```python
from build123d import *

# Parameters (mm, degrees)
SKETCH1_R           = 37.5
BOSS_EXTRUDE1_DEPTH = 10
SKETCH3_R           = 1.5
CUT_EXTRUDE3_DEPTH  = 54.967582862
SKETCH4_R           = 5
CUT_EXTRUDE4_DEPTH  = 5
SKETCH5_R           = 1.5
CUT_EXTRUDE5_DEPTH  = 54.967582862
SKETCH6_R           = 3
CUT_EXTRUDE6_DEPTH  = 5
SKETCH8_R           = 3
CUT_EXTRUDE7_DEPTH  = 3
SKETCH9_R           = 10
CUT_EXTRUDE8_DEPTH  = 54.967582862


with BuildPart() as part:
    # Sketch1 → Boss-Extrude1 (new body)
    with BuildSketch(Plane(origin=(0, 0, 0), x_dir=(1, 0, 0), z_dir=(0, 1, 0))):
        with Locations(Location((0, 0, 0), (0, 0, 270))):
            Circle(SKETCH1_R)
    extrude(amount=BOSS_EXTRUDE1_DEPTH)

    # Sketch3 → Cut-Extrude3 (cut, through all)
    with BuildSketch(Plane(origin=(0, 10, 0), x_dir=(1, 0, 0), z_dir=(0, 1, 0))):
        with Locations(Location((0, 0, 0), (0, 0, 270))):
            Circle(SKETCH3_R)
    extrude(amount=-CUT_EXTRUDE3_DEPTH, mode=Mode.SUBTRACT)

    # Sketch4 → Cut-Extrude4 (cut)
    with BuildSketch(Plane.XZ):
        with Locations(Location((0, 0, 0), (0, 0, 270))):
            Circle(SKETCH4_R)
    extrude(amount=-CUT_EXTRUDE4_DEPTH, mode=Mode.SUBTRACT)

    # Sketch5 → Cut-Extrude5 (cut, through all)
    with BuildSketch(Plane(origin=(0, 10, 0), x_dir=(1, 0, 0), z_dir=(0, 1, 0))):
        with BuildLine():
            ThreePointArc((-18.854509148, 24.228237343), (-21.625950603, 24.261294568), (-19.689620544, 22.278214534))
            Line((-19.689620544, 22.278214534), (-20.247076251, 23.670781637))
            Line((-20.247076251, 23.670781637), (-18.854509148, 24.228237343))
        make_face()
        with BuildLine():
            Line((-20.247076251, 23.670781637), (-19.689620544, 22.278214534))
            ThreePointArc((-19.689620544, 22.278214534), (-19.004863797, 22.830003295), (-18.747076251, 23.670781637))
            ThreePointArc((-18.747076251, 23.670781637), (-18.774179334, 23.954638419), (-18.854509148, 24.228237343))
            Line((-18.854509148, 24.228237343), (-20.247076251, 23.670781637))
        make_face()
        with BuildLine():
            ThreePointArc((-3.072081987, 30.546068688), (-2.270027815, 29.724650042), (-1.122059178, 29.710957292))
            Line((-1.122059178, 29.710957292), (-1.679514884, 31.103524394))
            Line((-1.679514884, 31.103524394), (-3.072081987, 30.546068688))
        make_face()
        with BuildLine():
            Line((-1.679514884, 31.103524394), (-1.122059178, 29.710957292))
            ThreePointArc((-1.122059178, 29.710957292), (-0.437302431, 30.262746053), (-0.179514884, 31.103524394))
            ThreePointArc((-0.179514884, 31.103524394), (-1.963371667, 32.576421311), (-3.072081987, 30.546068688))
            Line((-3.072081987, 30.546068688), (-1.679514884, 31.103524394))
        make_face()
        with Locations(Location((19.070534713, -20.910318461, 0), (0, 0, 270))):
            Circle(SKETCH5_R)
        with Locations(Location((0.564603471, -28.318390189, 0), (0, 0, 270))):
            Circle(SKETCH5_R)
    extrude(amount=-CUT_EXTRUDE5_DEPTH, mode=Mode.SUBTRACT)

    # Sketch6 → Cut-Extrude6 (cut)
    with BuildSketch(Plane.XZ):
        with Locations(Location((19.070534713, 20.910318461, 0), (0, 0, 270))):
            Circle(SKETCH6_R)
        with Locations(Location((0.564603471, 28.318390189, 0), (0, 0, 270))):
            Circle(SKETCH6_R)
        with Locations(Location((-1.679514884, -31.103524394, 0), (0, 0, 270))):
            Circle(SKETCH6_R)
        with Locations(Location((-20.247076251, -23.670781637, 0), (0, 0, 270))):
            Circle(SKETCH6_R)
    extrude(amount=-CUT_EXTRUDE6_DEPTH, mode=Mode.SUBTRACT)

    # Sketch8 → Cut-Extrude7 (cut)
    with BuildSketch(Plane(origin=(0, 10, 0), x_dir=(1, 0, 0), z_dir=(0, 1, 0))):
        with Locations(Location((0, 0, 0), (0, 0, 270))):
            Circle(SKETCH8_R)
    extrude(amount=-CUT_EXTRUDE7_DEPTH, mode=Mode.SUBTRACT)

    # Sketch9 → Cut-Extrude8 (cut, through all)
    with BuildSketch(Plane(origin=(0, 10, 0), x_dir=(1, 0, 0), z_dir=(0, 1, 0))):
        with Locations(Location((17.876448336, 6.629278922, 0), (0, 0, 270))):
            Circle(SKETCH9_R)
        with Locations(Location((-19.565700474, -7.94754173, 0), (0, 0, 270))):
            Circle(SKETCH9_R)
    extrude(amount=-CUT_EXTRUDE8_DEPTH, mode=Mode.SUBTRACT)


solid = part.part
```
Geometry: final body of the model. Coordinates: model frame, mm. A direction names the side the tool comes from. Round coordinates to 2 decimals unless told otherwise and drop trailing zeros. Write each loop counter-clockwise with the first axis right and the second up, starting at its lowest first coordinate (ties: lowest second). Pieces come first, ordered by that corner, then holes. Notation, with made-up numbers: (-16.5, 24.5) -> (20.5, 24.5) arc R30 ccw to (20.5, 55.5) -> close; hole circle Ø4 at (17, -34). An arc over 180 degrees is marked (long way). Use CSV: the item, a comma, the result in double quotes. Start each with the question number.
Q1. Line query: L1, parallel to Z at x = 0.5, y = 8; L2, parallel to X at y = 5.7, z = 0; L3, parallel to X at y = 7.65, z = 0. Output: solid intervals per line, ascending.
Q2. Reachability of faces 5 (the face through (20.335, 7.535, 21.717)), 6 (the face through (-4.88, 2.46, 1.08)), 7 (the face through (-1.3, 7, 1.3)) from +Z, -Z, +X, -X, +Y, -Y: full face, straight path, thin tool, end or side. Return the list, or none.
Q3. First-contact query: pin 1 Ø1.8 at (x, z) = (0.5, 0.5) entering from +Y; pin 2 Ø2.5 at (x, z) = (-20.25, -23.67) entering from +Y; pin 3 Ø1.8 at (x, z) = (-2.5, -30.5) entering from -Y; pin 4 Ø3 at (x, z) = (8.5, 4) entering from -Y. Flat tips, straight axial feed; report the tip coordinate or a pass-through.
Q4. Pull-direction query (X, two-part tool) for faces 1 (the face through (1.015, 7.535, 29.749)), 2 (the face through (-22.818, 4.93, -29.759)), 3 (the face through (0.697, 2.465, 31.315)), 4 (the face through (1, 0, 8)); classes: pulls with the +X half, pulls with the -X half, needs draft (parallel to the pull), parting line crosses it, or undercut.
Q5. Section D-D (z = 0). Return loops of the section in (x, y), plus the area to 3 significant figures.
Q6. Section C-C (y = 2.25). Return loops of the section in (x, z), plus the area to 3 significant figures.
Q7. Section B-B (x = -28). Return loops of the section in (y, z), plus the area to 3 significant figures.
Q8. Section A-A (z = 7.5). Return loops of the section in (x, y), plus the area to 3 significant figures.
Result sheet:
1,L1,"-37.5 to -2.96, 2.96 to 26.82, 29.82 to 37.5"
1,L2,"-37.5 to -25.64, -13.5 to -1.5, 1.5 to 10.39, 25.36 to 37.5"
1,L3,"-37.5 to -25.64, -13.5 to -3, 3 to 10.39, 25.36 to 37.5"
2,face 5,"+Y, -Y"
2,face 6,"-Y"
2,face 7,"+Y"
3,pin 1,"y = 7"
3,pin 2,"through"
3,pin 3,"y = 5"
3,pin 4,"y = 0"
4,face 1,"undercut"
4,face 2,"parting line crosses it"
4,face 3,"undercut"
4,face 4,"needs draft"
5,outline,"(-37.5, 0) -> (-25.64, 0) -> (-25.64, 10) -> (-37.5, 10) -> close; (-13.5, 0) -> (-5, 0) -> (-5, 5) -> (-1.5, 5) -> (-1.5, 7) -> (-3, 7) -> (-3, 10) -> (-13.5, 10) -> close; (1.5, 5) -> (5, 5) -> (5, 0) -> (10.39, 0) -> (10.39, 10) -> (3, 10) -> (3, 7) -> (1.5, 7) -> close; (25.36, 0) -> (37.5, 0) -> (37.5, 10) -> (25.36, 10) -> close"
5,area,"405 mm²"
6,outline,"circle Ø75 at (0, 0); hole circle Ø20 at (-19.57, 7.95); hole circle Ø6 at (-20.25, -23.67); hole circle Ø10 at (0, 0); hole circle Ø6 at (-1.68, -31.1); hole circle Ø6 at (0.56, 28.32); hole circle Ø20 at (17.88, -6.63); hole circle Ø6 at (19.07, 20.91)"
6,area,"3,600 mm²"
7,outline,"(0, -24.94) -> (10, -24.94) -> (10, 2.58) -> (0, 2.58) -> close; (0, 13.32) -> (10, 13.32) -> (10, 24.94) -> (0, 24.94) -> close"
7,area,"391 mm²"
8,outline,"(-36.74, 0) -> (-29.56, 0) -> (-29.56, 10) -> (-36.74, 10) -> close; (-9.58, 0) -> (36.74, 0) -> (36.74, 10) -> (-9.58, 10) -> close"
8,area,"535 mm²"
